Answer from the drawing. Dimensions are ordinates in mm from the lowest x, y and z of the part. Coordinates: 2 decimals unless noted, no trailing zeros. Order: outer loops, then holes, each group sorted by start corner. A loop starts at its lowest first (then second) coordinate and runs counter-clockwise, first axis right, second up. Notation, with made-up numbers: (-21, 66) -> (7, 66) arc R18 cw to (7, 72) -> close; hole circle Ø11 at (-25, 83). An arc over 180 degrees is marked (long way). Answer as a JSON object with one key per item and string values. Group by question number.
1) Section C-C on x = 2 is taken. Determine the outline of the cut face in (y, z).
2) Section A-A on y = 7.5 is taken. Determine the outline of the cut face in (x, z).
3) Section D-D on y = 3 is taken. Determine the outline of the cut face in (x, z).
4) Consider L1, parallel to X at y = 7.75, z = 1.25 (1 decimal); L2, parallel to X at y = 8.25, z = 9.75 (1 decimal); L3, parallel to Y at x = 5.75, z = 6.75. Determine where each line is inside the solid, lowest interval first.
5) Section B-B on z = 3.25 is taken. Determine the outline of the cut face in (x, y) (1 decimal).
6) Given pin 1 (1 mm diameter, centred on x = 4, z = 6, fed in from +Y) (1 decimal); pin 2 (4 mm diameter, centred on x = 2, z = 4.5, fed in from -Y), each flat-ended and moving along its own axis, determine where each tip first touches the part or whether it passes through.
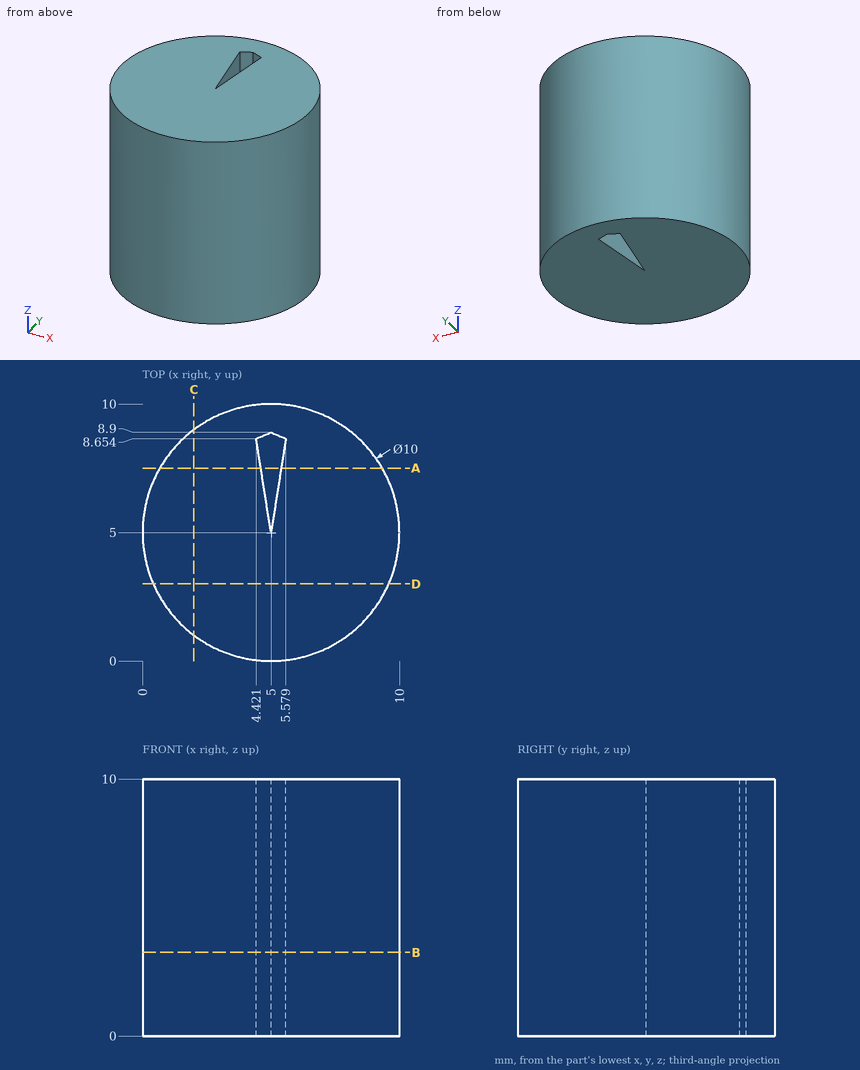
Worked answers:
{
 "1": {"outline": "(1, 0) -> (9, 0) -> (9, 10) -> (1, 10) -> close"},
 "2": {"outline": "(0.67, 0) -> (4.6, 0) -> (4.6, 10) -> (0.67, 10) -> close; (5.4, 0) -> (9.33, 0) -> (9.33, 10) -> (5.4, 10) -> close"},
 "3": {"outline": "(0.42, 0) -> (9.58, 0) -> (9.58, 10) -> (0.42, 10) -> close"},
 "4": {"L1": "x = 0.8 to 4.6, 5.4 to 9.2", "L2": "x = 1.2 to 4.5, 5.5 to 8.8", "L3": "y = 0.06 to 9.94"},
 "5": {"outline": "circle Ø10 at (5, 5); hole (4.4, 8.7) -> (5, 5) -> (5.6, 8.7) -> (5, 8.9) -> close"},
 "6": {"pin 1": "stops at y = 10", "pin 2": "stops at y = 0.1"}
}
